from build123d import *

# Parameters (mm, degrees)
SKETCH1_R           = 4.25
SKETCH1_R_2         = 3.75
SKETCH1_R_3         = 4.5
BOSS_EXTRUDE1_DEPTH = 6.5
CUT_EXTRUDE1_DEPTH  = 10
FILLET1_R           = 4.75
CHAMFER1_SIZE       = 1.5


with BuildPart() as part:
    # Sketch1 → Boss-Extrude1 (new body)
    with BuildSketch(Plane.XY):
        with BuildLine():
            Line((-11.458079381, -19.05), (53.381074139, -59.408818568))
            ThreePointArc((53.381074139, -59.408818568), (58.197626483, -59.528635467), (60.641156228, -55.376203052))
            Line((60.641156228, -55.376203052), (60.641156228, 14.3))
            ThreePointArc((60.641156228, 14.3), (59.249913439, 17.658757211), (55.891156228, 19.05))
            Line((55.891156228, 19.05), (-13.723477062, 19.05))
            ThreePointArc((-13.723477062, 19.05), (-14.628464695, 18.040083046), (-15.73121772, 18.829304583))
            ThreePointArc((-15.73121772, 18.829304583), (-17.658815789, 17.658815789), (-18.829304583, 15.73121772))
            ThreePointArc((-18.829304583, 15.73121772), (-18.040083046, 14.628464695), (-19.05, 13.723477062))
            Line((-19.05, 13.723477062), (-19.05, 8.996305235))
            ThreePointArc((-19.05, 8.996305235), (-18.034, 7.980305235), (-19.05, 6.964305235))
            Line((-19.05, 6.964305235), (-19.05, -6.964305235))
            ThreePointArc((-19.05, -6.964305235), (-18.034, -7.980305235), (-19.05, -8.996305235))
            Line((-19.05, -8.996305235), (-19.05, -13.723477062))
            ThreePointArc((-19.05, -13.723477062), (-18.040083046, -14.628464695), (-18.829304583, -15.73121772))
            ThreePointArc((-18.829304583, -15.73121772), (-17.658815789, -17.658815789), (-15.73121772, -18.829304583))
            ThreePointArc((-15.73121772, -18.829304583), (-14.628464695, -18.040083046), (-13.723477062, -19.05))
            Line((-13.723477062, -19.05), (-11.458079381, -19.05))
        make_face()
        with Locations(Location((41.314990606, -29.4594322, 0), (0, 0, 180))):
            Circle(SKETCH1_R, mode=Mode.SUBTRACT)
        with Locations(Location((41.591156228, 0, 0), (0, 0, 180))):
            Circle(SKETCH1_R_2, mode=Mode.SUBTRACT)
        with Locations(Location((0, 0, 0), (0, 0, 180))):
            Circle(SKETCH1_R_3, mode=Mode.SUBTRACT)
    extrude(amount=BOSS_EXTRUDE1_DEPTH)

    # Sketch3 → Cut-Extrude1 (cut)
    with BuildSketch(Plane(origin=(0, 0, 0), x_dir=(-1, 0, 0), z_dir=(0, 0, -1))):
        with BuildLine():
            Line((19.05, 6.964305235), (19.05, -6.964305235))
            Line((19.05, -6.964305235), (19.05, -13.723477062))
            Line((19.05, -13.723477062), (18.829304583, -15.73121772))
            ThreePointArc((18.829304583, -15.73121772), (17.658815789, -17.658815789), (15.73121772, -18.829304583))
            Line((15.73121772, -18.829304583), (13.723477062, -19.05))
            Line((13.723477062, -19.05), (11.458079381, -19.05))
            Line((11.458079381, -19.05), (-19.05, -38.039606954))
            Line((-19.05, -38.039606954), (-19.05, 8.996305235))
            Line((-19.05, 8.996305235), (-19.05, 13.723477062))
            Line((-19.05, 13.723477062), (-19.05, 19.05))
            Line((-19.05, 19.05), (13.723477062, 19.05))
            Line((13.723477062, 19.05), (15.73121772, 18.829304583))
            ThreePointArc((15.73121772, 18.829304583), (17.658815789, 17.658815789), (18.829304583, 15.73121772))
            Line((18.829304583, 15.73121772), (19.05, 13.723477062))
            Line((19.05, 13.723477062), (19.05, 6.964305235))
        make_face()
    extrude(amount=-CUT_EXTRUDE1_DEPTH, mode=Mode.SUBTRACT)

    # Fillet1
    fillet1_edges = [part.edges().sort_by_distance(p)[0] for p in [
        (19.05, -38.039606954, 3.25),
        (19.05, 19.05, 3.25),
    ]]
    fillet(fillet1_edges, radius=FILLET1_R)

    # Chamfer1
    chamfer1_edges = [part.edges().sort_by_distance(p)[0] for p in [
        (45.341156228, 0, 6.5),
        (45.564990606, -29.4594322, 6.5),
        (19.05, -10.550608772, 0),
        (20.441242789, 17.658757211, 0),
        (19.647567585, -37.707687799, 0),
        (19.05, -10.550608772, 6.5),
        (20.441242789, 17.658757211, 6.5),
        (19.647567585, -37.707687799, 6.5),
        (37.335496024, -49.421325814, 6.5),
        (45.564990606, -29.4594322, 0),
        (45.341156228, 0, 0),
        (58.197626483, -59.528635467, 6.5),
        (60.641156228, -20.538101526, 6.5),
        (39.845578114, 19.05, 0),
        (59.249913439, 17.658757211, 0),
        (60.641156228, -20.538101526, 0),
        (58.197626483, -59.528635467, 0),
        (37.335496024, -49.421325814, 0),
        (59.249913439, 17.658757211, 6.5),
        (39.845578114, 19.05, 6.5),
    ]]
    chamfer(chamfer1_edges, length=CHAMFER1_SIZE)


solid = part.part
Work out the finished part from the listing and answer in its coordinate system (mm). Coordinates: 2 decimals unless noted, no trailing zeros. Write each loop counter-clockwise with the first axis right and the second up, starting at its lowest first coordinate (ties: lowest second). Pieces come first, ordered by that corner, then holes. Notation, with made-up numbers: M 78.25,-22 L 126.25,-22 A14 ccw 126.25,0 Z; hole C 43,-39.5 d11. An arc over 180 degrees is marked long. Use one line per item in the form item = value. Start each with the question number.
1. The part is cut by section D-D (x = 25). Give the vertices of the cut face in (y, z), plus the area to 3 significant figures.
2. The mould has two halves that part along X. Classify faces 1 (the face through (44.45, -32.33, 3.23)), 2 (the face through (59.9, -21.03, 5.74)), 3 (the face through (19.79, -10.2, 5.74)): released by +X, released by -X, zero draft, split by the parting line, or undercut.
3. The part is cut by section A-A (y = 0). Give the vertices of the cut face in (x, z).
4. Straight lines are drawn through the part: probe 1 along Y at (x, z) = (45, 6); probe 2 along Y at (x, z) = (56, 3.25); probe 3 along Y at (x, z) = (39.5, 5.25). For each, find the intervals that lie inside material, in ascending order. Write a range as from..to.
5. Each of these flat-tipped pins is pushed along its axis until it touches: P1, Ø7, axis at x = 41.59, y = 0, coming from the -Z side; P2, Ø1.5, axis at x = 50.5, z = 4, coming from the -Y side. Where does it stop, or does it pass through?
6. The part is cut by section C-C (y = -13.5). Give the vertices of the cut face in (x, z), plus the area to 3 significant figures.
7. The part is cut by section B-B (z = 0.75). Give the vertices of the cut face in (x, y) (3 decimals).
Evaluation:
q1.outline = M -41.74,1.5 L -39.98,0 L 17.55,0 L 19.05,1.5 L 19.05,5 L 17.55,6.5 L -39.98,6.5 L -41.74,5 Z
q1.area = 390 mm^2
q2.face_1 = undercut
q2.face_2 = released by +X
q2.face_3 = released by -X
q3.outline = M 19.05,1.5 L 20.55,0 L 36.34,0 L 37.84,1.5 L 37.84,5 L 36.34,6.5 L 20.55,6.5 L 19.05,5 Z; M 45.34,1.5 L 46.84,0 L 59.14,0 L 60.64,1.5 L 60.64,5 L 59.14,6.5 L 46.84,6.5 L 45.34,5 Z
q4.probe_1 = -53.01..-33.2, -25.72..-3.31, 3.31..18.05
q4.probe_2 = -60.12..19.05
q4.probe_3 = -50.47..-33.58, -25.34..-3.41, 3.41..18.8
q5.P1 = through
q5.P2 = -58.08
q6.outline = M 19.05,1.5 L 20.55,0 L 59.14,0 L 60.64,1.5 L 60.64,5 L 59.14,6.5 L 20.55,6.5 L 19.05,5 Z
q6.area = 266 mm^2
q7.outline = M 19.8,-35.401 A4 ccw 21.686,-38.797 L 53.777,-58.772 A4 ccw 59.891,-55.376 L 59.891,14.3 A4 ccw 55.891,18.3 L 23.8,18.3 A4 ccw 19.8,14.3 Z; hole C 41.315,-29.459 d10; hole C 41.591,0 d9
